The listing builds one solid part. Answer for the finished solid, in the listing's coordinates (mm). Face numbers are marked on the shaded views. A direction names the side the tool comes from. Round coordinates to 2 decimals unless told otherwise and drop trailing zeros. Write each loop counter-clockwise with the first axis right and the second up, starting at its lowest first coordinate (ties: lowest second). Pieces come first, ordered by that corner, then holes. Notation, with made-up numbers: M 10.5,-5.5 L 38.5,-5.5 A24 cw 38.5,4.5 Z; hole C -34,79 d11. An arc over 180 degrees is marked long. Write each question's results on one line, items separated by ' | '.
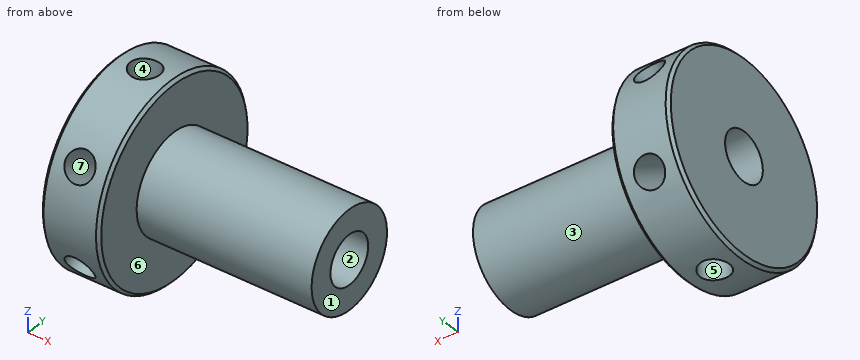
Autodesk Inventor part; units mm, degrees
ref_plane "Arbeitsebene1" through (0, 0, 10) normal (0, 0, 1) x (1, 0, 0)
ref_plane "YZ Plane" through (0, 0, 0) normal (1, 0, 0) x (0, 1, 0)
ref_plane "XZ Plane" through (0, 0, 0) normal (0, 1, 0) x (-1, 0, 0)
sketch "Skizze1" plane through (0, 0, 0) normal (0, 1, 0) x (-1, 0, 0)
  line L0 (0, 0) -> (0, 10)
  line L1 (0, 10) -> (-6, 10)
  line L2 (-6, 10) -> (-6, 5)
  line L3 (-6, 5) -> (-24, 5)
  line L4 (-24, 5) -> (-24, 0)
  line L5 (-24, 0) -> (0, 0)
  dimension "d0" = 20
  dimension "d1" = 10
  dimension "d2" = 6
  dimension "d3" = 18
revolve "Umdrehung1" add sketch "Skizze1" angle 360 about axis through (24, 0, 0) along (-1, 0, 0)
sketch "Skizze2" plane through (24, 0, 0) normal (1, 0, 0) x (0, 0, -1)
  circle A0 centre (0, 0) radius 5
hole "Bohrung1" at (24, 0, 0) direction (-1, 0, 0) diameter 5 depth 24
thread "Gewinde1"
ref_plane "Arbeitsebene1" through (0, 0, 10) normal (0, 0, 1) x (1, 0, 0)
sketch "Skizze3" plane through (0, 0, 10) normal (0, 0, 1) x (1, 0, 0)
  line L0 (0, 10) -> (0, -10)
  point P0 (0, 0)
  point P1 (3, 0)
  point P2 (0, 0)
  dimension "d15" = 3
hole "Bohrung2" at (3, 0, 10) direction (0, 0, -1) diameter 3 depth 6
pattern_circular "Runde Anordnung1" count 6 over 360 about axis through (3, 0, 0) along (-1, 0, 0) of "Bohrung2"
chamfer "Fasen1" distance 0.3 angle 45 2 edges at (0, 0, -10) (6, 0, -10)
properties part number "1153"
1) Section A-A (z = 0) is taken. Determine the outline of the cut face in (x, y), then the cut area to 3 significant figures.
Return value:
outline: M 0,-9.7 L 0.3,-10 L 5.7,-10 L 6,-9.7 L 6,-5 L 24,-5 L 24,-2.5 L 0,-2.5 Z; M 0,2.5 L 24,2.5 L 24,5 L 6,5 L 6,9.7 L 5.7,10 L 0.3,10 L 0,9.7 Z | area: 180 mm²
2) Each of these flat-tipped pins is pushed along its axis until it touches: pin 1 (1.5 mm diameter, centred on y = -4.5, z = 7, fed in from +X); pin 2 (10 mm diameter, centred on x = 6, z = -5.5, fed in from -Y); pin 3 (1.5 mm diameter, centred on x = 9.5, z = 3.5, fed in from +Y). Where does it stop, or does it pass through?
Return value:
pin 1: x = 6 | pin 2: y = -9.99 | pin 3: y = 4.18
3) Section D-D (x = 3) is taken. Determine the outline of the cut face in (y, z).
Return value:
outline: M -9.31,-3.64 L -4.21,-0.7 L -2.71,-3.3 L -7.81,-6.24 A10 ccw -1.5,-9.89 L -1.5,-4 L 1.5,-4 L 1.5,-9.89 A10 ccw 7.81,-6.24 L 2.71,-3.3 L 4.21,-0.7 L 9.31,-3.64 A10 ccw 9.31,3.64 L 4.21,0.7 L 2.71,3.3 L 7.81,6.24 A10 ccw 1.5,9.89 L 1.5,4 L -1.5,4 L -1.5,9.89 A10 ccw -7.81,6.24 L -2.71,3.3 L -4.21,0.7 L -9.31,3.64 A10 ccw Z; hole C 0,0 d5
4) A tool of negligible diameter and unlimited length cuts with its end or side. For the marked faces 4, 5, 6 and 7, from which of +Z, -Z, +X, -X, +Y, -Y can it reach the whole face along a straight path? Write none if from no direction.
Return value:
face 4: +Z | face 5: -Z | face 6: +X | face 7: none
5) The mould has two halves that part along Z. Classify the marked faces 1, 2 and 3: +Z half, -Z half, draft (parallel to the pull), parting line (faces both ways), or undercut.
Return value:
face 1: draft | face 2: undercut | face 3: parting line
6) Section B-B (y = 0) is taken. Determine the outline of the cut face in (x, z), then the cut area to 3 significant figures.
Return value:
outline: M 0,-9.7 L 0.3,-10 L 1.5,-10 L 1.5,-4 L 4.5,-4 L 4.5,-10 L 5.7,-10 L 6,-9.7 L 6,-5 L 24,-5 L 24,-2.5 L 0,-2.5 Z; M 0,2.5 L 24,2.5 L 24,5 L 6,5 L 6,9.7 L 5.7,10 L 4.5,10 L 4.5,4 L 1.5,4 L 1.5,10 L 0.3,10 L 0,9.7 Z | area: 144 mm²
7) Section C-C (x = 17) is taken. Determine the outline of the cut face in (y, z), then the cut area to 3 significant figures.
Return value:
outline: C 0,0 d10; hole C 0,0 d5 | area: 58.9 mm²
8) Find the intervals of material crossed by line 1 (X direction, y = 0, z = 6.75); line 2 (Y direction, x = 11.25, z = 0); line 3 (Z direction, x = 3.75, y = 6), in increasing order.
Return value:
line 1: 0 to 1.5, 4.5 to 6 | line 2: -5 to -2.5, 2.5 to 5 | line 3: -8 to -4.96, -1.96 to 1.96, 4.96 to 8
